from build123d import *

# Parameters (mm, degrees)
F0_R     = 127
F1_DEPTH = 114.3
F2_R     = 10
F3_R     = 6.35
F4_DEPTH = 114.3


with BuildPart() as f1:
    # F0 (on Right) → F1 (new body)
    with BuildSketch(Plane.YZ):
        Circle(F0_R)
    extrude(amount=-F1_DEPTH)

    # F2
    f2_edges = [f1.edges().sort_by_distance(p)[0] for p in [
        (0, -127, 0),
        (-114.3, -127, 0),
    ]]
    fillet(f2_edges, radius=F2_R)

    # F3 (on face) → F4 (cut, through all)
    with BuildSketch(Plane.YZ):
        Circle(F3_R)
    extrude(amount=-F4_DEPTH, mode=Mode.SUBTRACT)


solid = f1.part
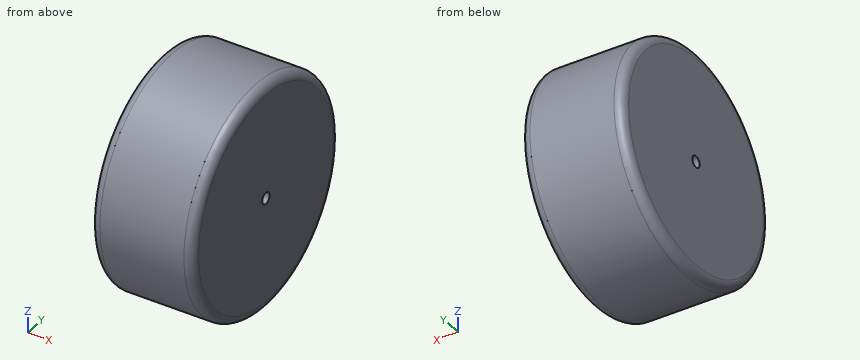
Design review of the part built by this model. Coordinates are the model's own, in mm. Round coordinates to 2 decimals unless told otherwise and drop trailing zeros. Loops run counter-clockwise (first coordinate to the right, second up) from the corner with the lowest first, then second, coordinate; pieces in that order, holes last. Notation, with made-up numbers: (0.5, 21) -> (33.5, 21) arc R27 cw to (33.5, 46) -> close; hole circle Ø5 at (86, -39). An arc over 180 degrees is marked (long way). Use one line per item in the form item = value. Start each with the question number.
Q1. Wall thickness on line 1 along Z through (x, y) = (-60, 0); line 2 along Z through (x, y) = (-37.5, 10); line 3 along Y through (x, z) = (-51, -106): over which ranges is each line inside the solid? List them lowest first. Write a range as [from, to].
Q2. We need section A-A on y = 0. Give the boundary of the cut face in (x, z).
Q3. We need section C-C on x = -41. Give the boundary of the cut face in (y, z).
Q4. For pin 1 Ø3 at (x, z) = (-94, 79) entering from +Y; pin 2 Ø10 at (x, y) = (-81, -54) entering from -Z; pin 3 Ø6 at (x, z) = (-34.5, -22) entering from +Y, all flat-tipped, find the tip position at first contact; note any pin that passes through.
Calculated:
q1.line_1 = [-127, -6.35], [6.35, 127]
q1.line_2 = [-126.61, 126.61]
q1.line_3 = [-69.95, 69.95]
q2.outline = (-114.3, -117) arc R10 ccw to (-104.3, -127) -> (-10, -127) arc R10 ccw to (0, -117) -> (0, -6.35) -> (-114.3, -6.35) -> close; (-114.3, 6.35) -> (0, 6.35) -> (0, 117) arc R10 ccw to (-10, 127) -> (-104.3, 127) arc R10 ccw to (-114.3, 117) -> close
q3.outline = circle Ø254 at (0, 0); hole circle Ø12.7 at (0, 0)
q4.pin_1 = 100.61
q4.pin_2 = -117.17
q4.pin_3 = 125.57
